Autodesk Inventor part; units mm, degrees
ref_plane "YZ Plane" through (0, 0, 0) normal (1, 0, 0) x (0, 1, 0)
ref_plane "XZ Plane" through (0, 0, 0) normal (0, 1, 0) x (-1, 0, 0)
ref_plane "XY Plane" through (0, 0, 0) normal (0, 0, 1) x (1, 0, 0)
sketch "Sketch1" plane through (0, 0, 0) normal (0, 0, 1) x (1, 0, 0)
  line L0 (0, 0) -> (-320, 0)
  line L1 (0, -94) -> (0, 0)
  line L2 (-320, 0) -> (-320, -70)
  line L3 (-320, -70) -> (0, -94)
  point P0 (0, -47)
  dimension "d32" = 94
  dimension "d60" = 70
  dimension "d61" = 320
extrude "Plate1" add sketch "Sketch1" along normal blind 2
sketch "Sketch8" plane through (0, 0, 2) normal (0, 0, 1) x (1, 0, 0)
  line L0 (-29.75, -53.25) -> (-60.25, -53.25)
  line L1 (-60.25, -53.25) -> (-60.25, -22.75)
  line L2 (-60.25, -22.75) -> (-29.75, -22.75)
  line L3 (-29.75, -22.75) -> (-29.75, -53.25)
  line L4 (-29.75, -53.25) -> (-60.25, -22.75) construction
  line L5 (-60.25, -53.25) -> (-29.75, -22.75) construction
  circle A0 centre (-22, -61) radius 2.5
  circle A1 centre (-68, -61) radius 2.5
  circle A2 centre (-68, -15) radius 2.5
  circle A3 centre (-22, -15) radius 2.5
  line L6 (0, 0) -> (0, -94)
  line L7 (-320, 0) -> (0, 0)
  line L8 (-60.25, -53.25) -> (-68, -61) construction
  line L9 (-68, -15) -> (-22, -15) construction
  line L10 (-22, -15) -> (-22, -61) construction
  line L11 (-22, -61) -> (-68, -61) construction
  line L12 (-68, -61) -> (-68, -15) construction
  point P0 (-45, -38)
  dimension "d51" = 30.5
  dimension "d52" = 30.5
  dimension "d53" = 5
  dimension "d72" = 45
  dimension "d78" = 46
  dimension "d79" = 15
extrude "Cut3" cut sketch "Sketch8" against normal blind 2
pattern_linear "Rectangular Pattern1" count 3 spacing 120 along (-1, 0, 0) of "Cut3"
sketch "Sketch9" plane through (0, -2, 2) normal (0, 1, 0) x (-1, 0, 0)
  line L0 (320, 0) -> (0, 0)
  line L1 (0, 0) -> (0, -72)
  line L2 (0, -72) -> (320, -72)
  line L3 (320, -72) -> (320, 0)
edge flange "Flange3" height 72 angle 90 thickness 2 bend radius 2.75 thickness toward (0, 1, 0) relief round relief width 2 relief depth 1 edges at (-160, 0, 0) wall of the first edge with corners at (-320, -2, 2) (0, -2, 2) (0, -2, -70) (-320, -2, -70)
bend "Bend3"
corner "Corner3"
equation "\"d51\" = d52"
equation "\"d55\" = Thickness"
equation "\"d2\" = Thickness"
equation "\"d62\" = BendReliefWidth"
equation "\"d63\" = BendReliefDepth"
equation "\"d64\" = MinimumRemnant"
equation "\"d65\" = TransitionRadius"
equation "\"d68\" = BendRadius"
equation "\"d69\" = CornerReliefSize"
equation "\"d70\" = GapSize"
equation "\"d71\" = JacobiRadiusSize"
equation "\"BendReliefWidth\" = Thickness"
equation "\"BendReliefDepth\" = 0.5 * Thickness"
equation "\"CornerReliefSize\" = 4 * Thickness"
equation "\"MinimumRemnant\" = 2 * Thickness"
equation "\"TransitionRadius\" = BendRadius"
equation "\"JacobiRadiusSize\" = BendRadius"
equation "\"GapSize\" = Thickness"
properties part number "PRS 8422 BOTTOM FDS diameter way up_940" material "Stainless Steel"
Part model, mm, in its own coordinate system. A direction names the side the tool comes from. Coordinates: 2 decimals unless noted, no trailing zeros. Loops run counter-clockwise (first coordinate to the right, second up) from the corner with the lowest first, then second, coordinate; pieces in that order, holes last. Notation, with made-up numbers: M -30,28 L 15,28 A13 ccw 15,38 Z; hole C 72.5,73.5 d4. An arc over 180 degrees is marked long. Use a Markdown table: item, result. Add a question column.
Q1. Cut at C-C (z = -17). Write the cut outline in (x, y).
Q2. Cut at B-B (y = -8.5). Write the cut outline in (x, z).
Q3. Probe L1, parallel to Y at x = -308, z = 0.7; L2, parallel to Y at x = -262, z = 0.4; L3, parallel to Y at x = -192.5, z = -52. List the from-to ranges inside material, lowest first.
Q4. Pin check, flat tips, straight feed: P1, Ø4, axis at x = -285.5, z = -43, coming from the -Y side; P2, Ø0.6, axis at x = -43.5, z = 0.5, coming from the -Y side; P3, Ø5, axis at x = -158.5, y = -84.5, coming from the -Z side. Stop position of each tip, or through.
Q5. Which spindle directions (+Z, -Z, +X, -X, +Y, -Y) get a long thin tool onto all of the face, cutting with end or side? Do faces 1 (the flat face through (-158, -2, -36)), 2 (the flat face through (-158, 0, -37)). Say none if no direction does.
Q6. Cut at A-A (x = -208.5). Write the cut outline in (y, z), and give its area (3 significant figures).
Worked out:
| question | item | result |
|---|---|---|
| 1 | outline | M -320,-2 L 0,-2 L 0,0 L -320,0 Z |
| 2 | outline | M -320,0 L 0,0 L 0,2 L -320,2 Z |
| 3 | L1 | y = -70.9 to -63.5, -58.5 to -17.5, -12.5 to -1.49 |
| 3 | L2 | y = -74.35 to -63.5, -58.5 to -17.5, -12.5 to -1.19 |
| 3 | L3 | y = -2 to 0 |
| 4 | P1 | stops at y = -2 |
| 4 | P2 | stops at y = -90.76 |
| 4 | P3 | stops at z = 0 |
| 5 | face 1 | -Z, +X, -X, -Y |
| 5 | face 2 | +Z, -Z, +X, -X, +Y |
| 6 | outline | M -78.36,0 L -4.75,0 A2.75 cw -2,-2.75 L -2,-70 L 0,-70 L 0,-2.75 A4.75 ccw -4.75,2 L -78.36,2 Z |
| 6 | area | 294 mm2 |
